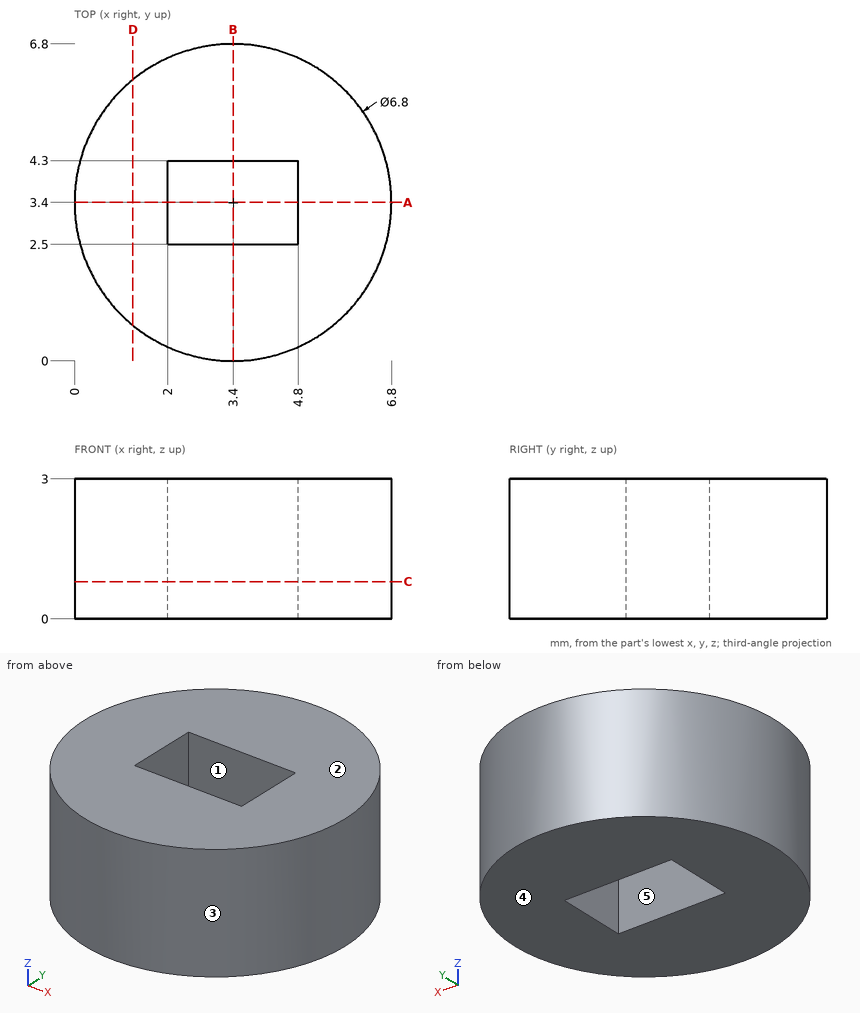
Input: dimensioned drawing with shaded views. Units: mm. Origin: part minimum x, y, z. A direction names the side the tool comes from. Round coordinates to 2 decimals unless told otherwise and drop trailing zeros. Order: outer loops, then holes, each group sorted by start corner. A loop starts at its lowest first (then second) coordinate and runs counter-clockwise, first axis right, second up. Notation, with made-up numbers: (0.5, 56) -> (50.5, 56) arc R34 cw to (50.5, 88) -> close; hole circle Ø1 at (-31.75, -23). An arc over 180 degrees is marked (long way). One line per item, written item: value. Start each with the question number.
Q1. Section query D-D (x = 1.25). Return the cut outline in (y, z).
Q2. Draft query along X for the marked faces 1, 2 and 3. Return one class per face: pulls with the +X half, pulls with the -X half, needs draft (parallel to the pull), parting line crosses it, or undercut.
Q3. Access query for the marked faces 4 and 5. Directions: +Z, -Z, +X, -X, +Y, -Y. A direction counts if a zero-diameter tool reaches every point of the face in a straight line with its end or side. Return the directions, or none.
Q4. Section query B-B (x = 3.4). Return the cut outline in (y, z).
Q5. Pin query (flat end, axial travel): pin 1 (1.5 mm diameter, centred on x = 2.5, z = 1, fed in from -Y). Return the tip coordinate at first contact, or that it passes through.
Q6. Section query A-A (y = 3.4). Return the cut outline in (x, z).
Q7. Section query C-C (z = 0.8). Return the cut outline in (x, y), plus the area to 3 significant figures.
Q8. Material intervals for probe 1 along X at (y, z) = (3.5, 2); probe 2 along Y at (x, z) = (2.5, 2.6); probe 3 along Y at (x, z) = (3.75, 2.7), sorted ascending.
Findings below:
1. outline: (0.77, 0) -> (6.03, 0) -> (6.03, 3) -> (0.77, 3) -> close
2. face 1: undercut
2. face 2: needs draft
2. face 3: parting line crosses it
3. face 4: -Z, +X, -X, +Y, -Y
3. face 5: +Z, -Z
4. outline: (0, 0) -> (2.5, 0) -> (2.5, 3) -> (0, 3) -> close; (4.3, 0) -> (6.8, 0) -> (6.8, 3) -> (4.3, 3) -> close
5. pin 1: y = 0
6. outline: (0, 0) -> (2, 0) -> (2, 3) -> (0, 3) -> close; (4.8, 0) -> (6.8, 0) -> (6.8, 3) -> (4.8, 3) -> close
7. outline: circle Ø6.8 at (3.4, 3.4); hole (2, 2.5) -> (4.8, 2.5) -> (4.8, 4.3) -> (2, 4.3) -> close
7. area: 31.3 mm²
8. probe 1: 0 to 2, 4.8 to 6.8
8. probe 2: 0.12 to 2.5, 4.3 to 6.68
8. probe 3: 0.02 to 2.5, 4.3 to 6.78
